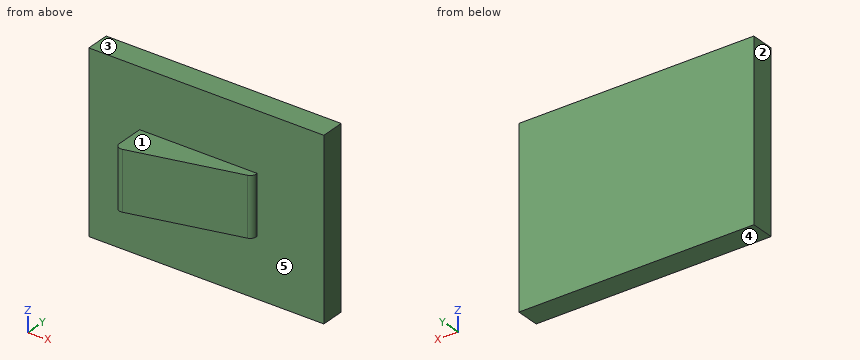
Solid Edge part; units mm, degrees
sketch "Sketch1" plane through (0, 0, 0) normal (0, -1, 0) x (1, 0, 0)
  line L0 (10.6791, 7.5) -> (-9.3209, 7.5)
  line L1 (-9.3209, 7.5) -> (-9.3209, -7.5)
  line L2 (-9.3209, -7.5) -> (10.6791, -7.5)
  line L3 (10.6791, -7.5) -> (10.6791, 7.5)
extrude "Protrusion1" add sketch "Sketch1" against normal blind 2
sketch "Sketch2" plane through (0.6791, 0, 0) normal (0, -1, 0) x (1, 0, 0)
  line L0 (4.3209, 2.5) -> (-5.6791, 2.5)
  line L1 (-5.6791, 2.5) -> (-5.6791, -2.5)
  line L2 (-5.6791, -2.5) -> (4.3209, -2.5)
  line L3 (4.3209, -2.5) -> (4.3209, 2.5)
extrude "ExtrudedProtrusion_2" add sketch "Sketch2" along normal blind 3
sketch "Sketch3" plane through (0, -1.5, -2.5) normal (0, 0, -1) x (1, 0, 0)
  line L0 (5, 1.5) -> (5, -1)
  line L1 (5, -1) -> (-5, 1.5)
  line L2 (-5, 1.5) -> (5, 1.5)
extrude "ExtrudedCutout_2" cut sketch "Sketch3" against normal blind 5
fillet "Round_2" radius 0.5 2 edges at (-5, -3, 0) (5, -0.5, 0)
Geometry: final body of the model. Coordinates: model frame, mm. Face numbers are marked on the shaded views. A direction names the side the tool comes from. Give positions to 0.01 mm unless a question says otherwise; leave off trailing zeros. Write each loop counter-clockwise with the first axis right and the second up, starting at its lowest first coordinate (ties: lowest second). Pieces come first, ordered by that corner, then holes.
1. Section query C-C, the plane y = -1.25. Return loops of the section in (x, z).
2. Line query: probe 1 along Y at (x, z) = (7.5, -1.75); probe 2 along Z at (x, y) = (-2.75, -1.9); probe 3 along Y at (x, z) = (-2, -1). Output: solid intervals per line, ascending.
3. Section query A-A, the plane z = 0.25. Return loops of the section in (x, y), then the cut area to 3 significant figures.
4. Pin query (flat end, axial travel): P1, Ø0.9, axis at x = 1.5, y = -1.5, coming from the +Z side; P2, Ø7.5, axis at x = 0, z = -3.5, coming from the -Y side; P3, Ø1.5, axis at x = 3.5, y = -1, coming from the -Z side. Return the tip coordinate at first contact, or that it passes through.
5. Reachability of the marked faces 1 and 2 from +Z, -Z, +X, -X, +Y, -Y: full face, straight path, thin tool, end or side. Return the list, or none.
6. Draft query along Z for the marked faces 3, 4 and 5. Return one class per face: released by +Z, released by -Z, zero draft, split by the parting line, or undercut.
7. Section query B-B, the plane x = 6.25. Return loops of the section in (y, z), then the cut area to 3 significant figures.
Computed:
1. outline: (-5, -2.5) - (2, -2.5) - (2, 2.5) - (-5, 2.5) - close
2. probe 1: y = 0 to 2
2. probe 2: z = -2.5 to 2.5
2. probe 3: y = -2.25 to 2
3. outline: (-9.32, 0) - (-5, 0) - (-5, -2.36) arc R0.5 ccw to (-4.38, -2.84) - (4.62, -0.59) arc R0.5 ccw to (5, -0.11) - (5, 0) - (10.68, 0) - (10.68, 2) - (-9.32, 2) - close
3. area: 57.4 mm2
4. P1: stops at z = 2.5
4. P2: stops at y = -2.65
4. P3: stops at z = -2.5
5. face 1: +Z, +X, -X, -Y
5. face 2: +Z, -Z, -X, +Y, -Y
6. face 3: released by +Z
6. face 4: released by -Z
6. face 5: zero draft
7. outline: (0, -7.5) - (2, -7.5) - (2, 7.5) - (0, 7.5) - close
7. area: 30.0 mm2
